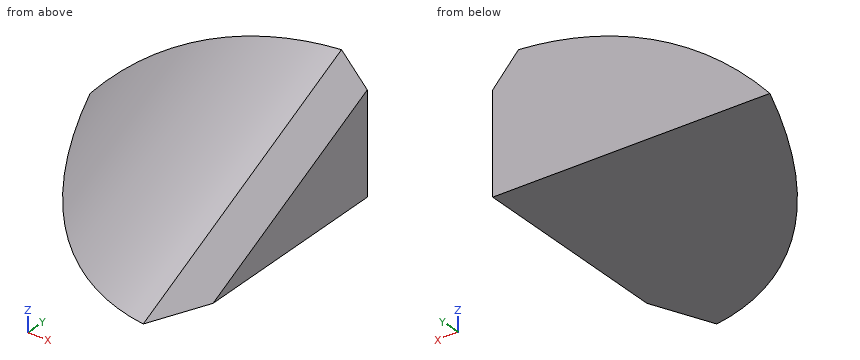
from build123d import *

# Parameters (mm, degrees)
F3_DEPTH    = 76.2
F4_SIZE     = 5.08
F5_T1_DEPTH = 438.8719745558


# Not quite as in the source:
# - a fillet or chamfer that OpenCascade refuses, or shapes differently, is made with other operations: its cross-section is extruded or revolved along the edge and cut away or added
# - a feature of the source that left no trace in its solid (it failed there, or was rolled back) is left out


with BuildPart() as f3:
    # F2 (on Right) → F3 (new body)
    with BuildSketch(Plane.YZ):
        Polygon((-52.9574006796, 0), (0, 0), (0, 25.36736615), align=None)
    extrude(amount=-F3_DEPTH)

    # F4
    f4_edges = [f3.edges().sort_by_distance(p)[0] for p in [
        (0, -26.4787, 12.683683),
    ]]
    chamfer(f4_edges, length=F4_SIZE)

    # F5: fillet of radius 76.2 on 1 edges, made by hand

    # F5_s2 → F5_t1 (cut)
    with BuildSketch(Plane(origin=(0, 181.3074352717, 86.8489018954), x_dir=(1, 0, 0), z_dir=(0, -0.9018694789, -0.4320086144))):
        with BuildLine():
            ThreePointArc((-5.08, 22.8780532919), (-55.6486118425, -1.0979149163), (-76.2, -53.1524248074))
            Line((-76.2, -53.1524248074), (-76.2, 22.8780532919))
            Line((-76.2, 22.8780532919), (-5.08, 22.8780532919))
        make_face()
    extrude(amount=F5_T1_DEPTH, mode=Mode.SUBTRACT)


solid = f3.part
Read the model definition and answer for the solid it produces. Units are mm, in the model's axes. Round coordinates to 2 decimals unless told otherwise and drop trailing zeros. Order: outer loops, then holes, each group sorted by start corner. A loop starts at its lowest first (then second) coordinate and runs counter-clockwise, first axis right, second up.
1) Straight lines are drawn through the part: L1, parallel to X at y = -2.5, z = 3.5; L2, parallel to Y at x = -4.5, z = 18.5; L3, parallel to Z at x = -28, y = -39. For each, find the intervals that lie inside material, in ascending order.
2) The part is cut by section A-A on x = -43.5. Write down the section's boundary in (y, z), plus the area to 3 significant figures.
3) The part is cut by section B-B on x = -16.5. Write down the section's boundary in (y, z), plus the area to 3 significant figures.
4) Flat-ended cylindrical pins translate along their axes: pin 1 (1.5 mm diameter, centred on x = -10, y = -12, fed in from +Z); pin 2 (5 mm diameter, centred on y = -12.5, z = 12.5, fed in from -X); pin 3 (12 mm diameter, centred on y = -30.5, z = 14.5, fed in from +X). Find the tip coordinate at first contact, or state that the pin passes through.
Resolved:
1. L1: x = -50.13 to 0
1. L2: y = -12.99 to 0
1. L3: z = 0 to 0.96
2. outline: (-21.78, 0) - (0, 0) - (0, 10.44) - close
2. area: 114 mm2
3. outline: (-49.17, 0) - (0, 0) - (0, 23.55) - close
3. area: 579 mm2
4. pin 1: stops at z = 19.45
4. pin 2: stops at x = -35.69
4. pin 3: stops at x = -2.46
